Part model, mm, in its own coordinate system. Coordinates: 2 decimals unless noted, no trailing zeros. Loops run counter-clockwise (first coordinate to the right, second up) from the corner with the lowest first, then second, coordinate; pieces in that order, holes last. Notation, with made-up numbers: (34.25, -36) - (91.25, -36) arc R21 ccw to (91.25, -29) - close; hole circle Ø7 at (-22, 25). An arc over 180 degrees is marked (long way). Use a Markdown table: item, result. Add a question column.
1. Band-saw the part on A-A, the plane x = -32.5. Give the cut face in (y, z) (3 decimals), plus the area to 3 significant figures.
2. Drop flat-ended pins along their axis: pin 1 (4 mm diameter, centred on x = 17, y = 32, fed in from +Z); pin 2 (10 mm diameter, centred on y = 40.5, z = 55.5, fed in from +X); pin 3 (5 mm diameter, centred on y = 36.5, z = 16.5, fed in from +X). Give the stop position or say it passes through.
3. Band-saw the part on B-B, the plane z = 51.5. Give the cut face in (x, y).
4. Wall check: probe 1 along Z at (x, y) = (-6.5, 30.5) (3 decimals); probe 2 along Z at (x, y) = (-5, 29) (3 decimals); probe 3 along Z at (x, y) = (19, 12) (3 decimals). Give the ranges that are in metal, low to high. Write a range as [from, to].
5. Pull direction Z, two halves, no side cores. Call faces 1 (the cylindrical face through (26.855, 44.028, 1.702)), 2 (the flat face through (11.015, 42.318, 25.785)), 3 (the flat face through (-1, 35, 0)): pulls with the +Z half, pulls with the -Z half, needs draft (parallel to the pull), parting line crosses it, or undercut.
from build123d import *

# Parameters (mm, degrees)
F1_DEPTH    = 3.175
F5_DEPTH    = 3.175
F6_T1_DEPTH = 117.475
F8_DEPTH    = 3.175


# Not quite as in the source:
# - a fillet or chamfer that OpenCascade refuses, or shapes differently, is made with other operations: its cross-section is extruded or revolved along the edge and cut away or added


with BuildPart() as f1:
    # F0 (on Top) → F1 (new body)
    with BuildSketch(Plane.XY):
        Polygon((50.8, 0), (0, 87.9881810245), (-50.8, 0), align=None)
    extrude(amount=F1_DEPTH)

    # F4 (on line) → F5 (join)
    with BuildSketch(Plane(origin=(30.2473107364, 17.7959839325, 17.4632910558), x_dir=(-0.3931673168, 0.8910065242, -0.226995231), z_dir=(0.7716343063, 0.4539904997, 0.445503225))):
        Polygon((6.5029600393, 75.2459340132), (-19.9755570322, -25.4006840255), (78.3980433443, 0), align=None)
    extrude(amount=F5_DEPTH)

    # F6: fillet of radius 3.175 on 1 edges, made by hand

    # F6_s2 → F6_t1 (cut)
    with BuildSketch(Plane(origin=(17.005719551, -29.012184774, 0.1101218851), x_dir=(-0.862716434, -0.5056880012, 0), z_dir=(-0.5056852899, 0.8627118085, -0.0032746052))):
        with BuildLine():
            ThreePointArc((-45.25402581, 4.1728704395), (-45.421662158, 1.7486197382), (-43.8259948462, -0.0841211704))
            Line((-43.8259948462, -0.0841211704), (-46.668506133, 1.3303591527))
            Line((-46.668506133, 1.3303591527), (-45.25402581, 4.1728704395))
        make_face()
    extrude(amount=F6_T1_DEPTH, mode=Mode.SUBTRACT)

    # F7 (on face) → F8 (cut, through all)
    with BuildSketch(Plane(origin=(32.697249659, 19.2374037692, 18.877763795), x_dir=(-0.3931673168, 0.8910065242, -0.226995231), z_dir=(0.7716343063, 0.4539904997, 0.445503225))):
        with BuildLine():
            ThreePointArc((23.2165575735, 13.9849704437), (26.5917627129, 16.2568894847), (27.8951978201, 20.1110668007))
            ThreePointArc((27.8951978201, 20.1110668007), (25.399375136, 25.1576316934), (19.8738380667, 26.2371631576))
            Line((19.8738380667, 26.2371631576), (23.2165575735, 13.9849704437))
        make_face()
        with BuildLine():
            Line((23.2165575735, 13.9849704437), (19.8738380667, 26.2371631576))
            ThreePointArc((19.8738380667, 26.2371631576), (15.4191014631, 18.4397070472), (23.2165575735, 13.9849704437))
        make_face()
    extrude(amount=-F8_DEPTH, mode=Mode.SUBTRACT)


solid = f1.part
Geometry check:
| question | item | result |
|---|---|---|
| 1 | outline | (0, 0) - (31.697, 0) - (31.697, 3.175) - (0, 3.175) - close |
| 1 | area | 101 mm^2 |
| 2 | pin 1 | stops at z = 37.08 |
| 2 | pin 2 | stops at x = 3.17 |
| 2 | pin 3 | stops at x = 25.97 |
| 3 | outline | (-6.53, 46.9) - (12.26, 14.97) - (15.77, 16) - (-3.92, 49.45) - close |
| 4 | probe 1 | z = [0, 3.175], [68.165, 75.292] |
| 4 | probe 2 | z = [0, 3.175], [67.096, 74.223] |
| 4 | probe 3 | z = [0, 3.175] |
| 5 | face 1 | parting line crosses it |
| 5 | face 2 | undercut |
| 5 | face 3 | pulls with the -Z half |
